Could you check a few things on this model? Use its own coordinates, in mm. Face numbers are marked on the shaded views. A direction names the side the tool comes from. Coordinates: 2 decimals unless noted, no trailing zeros. Write each loop counter-clockwise with the first axis right and the second up, starting at its lowest first coordinate (ties: lowest second). Pieces come first, ordered by that corner, then holes. Notation, with made-up numbers: (31, 57) - (71, 57) arc R27 ccw to (71, 82) - close; hole circle Ø7 at (77.5, 48). An arc over 180 degrees is marked (long way). Answer as a JSON object with one key per item and string values. Group by question number.
1) If we section it at C-C (x = -1.75): Write out the boundary of the cut face in (y, z).
2) On a 3-axis mill with a long thin cutter (end or side, diameter ignored), from which of +Z, -Z, +X, -X, +Y, -Y can I reach the whole of each face in a straight line? I mean the marked faces 1, 2, 3, 4 and 5. Say none if no direction works.
3) If we section it at D-D (y = 10.5): Write out the boundary of the cut face in (x, z).
4) If we section it at A-A (y = 8): Write out the boundary of the cut face in (x, z), plus the area to 3 significant figures.
5) We'd pull the mould along X, two halves only. Please class the marked faces 6, 7, 8 and 9: released by +X, released by -X, zero draft, split by the parting line, or undercut.
6) Will these pins go through, and if not, where does the flat tip stop? pin 1 Ø3 at (y, z) = (8, 0) entering from +X; pin 2 Ø6.5 at (y, z) = (6.5, 1) entering from +X; pin 3 Ø0.6 at (y, z) = (5.5, 7.5) entering from -X; pin 4 Ø4.5 at (y, z) = (-1.5, -1.5) entering from +X.
7) Please list where these lines run through material, in increasing order: line 1 along Y through (x, z) = (-14.05, 0); line 2 along X through (y, z) = (15.5, 7.5); line 3 along Z through (x, y) = (-11.8, 8).
8) If we section it at B-B (z = 0): Write out the boundary of the cut face in (x, y), plus the area to 3 significant figures.
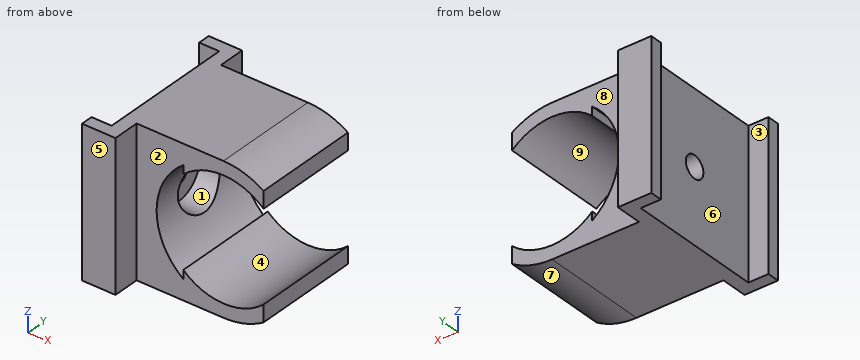
Autodesk Fusion 360 part; units mm, degrees
cylinder "CylinderPrimitive1" add diameter 18.5 height 80 placed x (1, 0, 0) y (0, 0, -1) z (0, 1, 0) at (0, 0, 0) makes body 1
sketch "Sketch2" plane through (0, 0, 0) normal (0, 1, 0) x (1, 0, 0)
  circle A0 centre (0, 0) radius 9
  line L0 (-23.395, 11) -> (16.2834, 11)
  line L1 (16.2834, 11) -> (16.2834, -11)
  line L2 (16.2834, -11) -> (-23.395, -11)
  line L3 (-23.395, -11) -> (-23.395, 11)
  circle A1 centre (0, 0) radius 10
  line L4 (0, 17.0641) -> (0, -18.6824) construction
  line L5 (-36.3056, 0) -> (26.2246, 0) construction
  line L6 (0, 9) -> (13.2349, 9)
  line L7 (13.2349, 9) -> (13.2349, -9)
  line L8 (13.2349, -9) -> (0, -9)
  line L9 (0, -9) -> (0, 9)
  line L10 (6, 8) -> (6, -8)
  circle A2 centre (0, 0) radius 11
  line L11 (6, 8) -> (6, 11)
  line L12 (6, -8) -> (6, -11)
  line L13 (-13, 11) -> (-18, 11)
  line L14 (-18, 11) -> (-18, -11)
  line L15 (-18, -11) -> (-13, -11)
  line L16 (-13, -11) -> (-13, 11)
  line L17 (-6, 8) -> (-6, -8)
  line L18 (-6, -8) -> (-6, -11)
  line L19 (-6, 8) -> (-6, 11)
  dimension "d3" = 18
  dimension "d4" = 11
  dimension "d5" = 11
  dimension "d6" = 1
  dimension "d7" = 6
  dimension "d8" = 2
  dimension "d9" = 5
  dimension "d10" = 13
extrude "Extrude1" add sketch "Sketch2" along normal blind 16 separate body contours A0 A1 L6 L10 | A0 A1 L8 L10 | A0 A1 L6 L17 | A1 L6 L11 | A0 A1 L8 L17 | A1 L8 L12 | A1 L6 A2 L11 L19 | A1 L8 A2 L12 L18 | A1 A2 L18 L19 | L0 A2 L19 | L0 L2 A2 L16 L18 L19 | L2 A2 L18 | L0 L2 L13 L14 L15 L16 makes body 2
sketch "Sketch3" plane through (-18, 0, 0) normal (-1, 0, 0) x (0, 0, 1)
  line L0 (-11, 0) -> (11, 0)
  line L1 (11, 0) -> (11, 16)
  line L2 (11, 16) -> (-11, 16)
  line L3 (-11, 16) -> (-11, 0)
  line L4 (11, 16) -> (-11, 0)
  line L5 (-11, 16) -> (11, 0)
  line L6 (-14, 18.2) -> (14, 18.2)
  line L7 (14, 18.2) -> (14, -2.2)
  line L8 (14, -2.2) -> (-14, -2.2)
  line L9 (-14, -2.2) -> (-14, 18.2)
  point P0 (0, 8)
  dimension "d21" = 10.2
  dimension "d22" = 10.2
  dimension "d23" = 14
  dimension "d24" = 14
hole "Hole1" at (-18, 8, 0) direction (1, 0, 0) diameter 3.332 end through all bodies 1 2
extrude "Extrude2" add sketch "Sketch2" along normal blind 20 and the other way blind 4 contours L0 L2 L13 L14 L15 L16 bodies 2
extrude "Extrude3" cut sketch "Sketch3" against normal blind 3 contours L0 L4 L5 | L3 L4 L5 | L1 L4 L5 | L2 L4 L5 | L6 L7 L8 L9 bodies 2
hole "Hole2" at (-18, 8, 0) direction (1, 0, 0) diameter 3.332 end through all bodies 1 2
ref_plane "WorkPlane1" through (-9, 0, 0) normal (1, 0, 0) x (0, 1, 0)
sketch "Sketch4" plane through (-9, 0, 0) normal (1, 0, 0) x (0, 0, -1)
  point P0 (0, 8)
hole "Hole3" at (-9, 8, 0) direction (-1, 0, 0) diameter 8 depth 4 tip angle 180 bodies 2
hidden bodies 1
Here are the results:
{
 "1": {"outline": "(0, -11) - (16, -11) - (16, -8.83) - (0, -8.83) - close; (0, 8.83) - (16, 8.83) - (16, 11) - (0, 11) - close"},
 "2": {"face 1": "+X", "face 2": "+Z, -Z, +X, -Y", "face 3": "+Z, -Z, -X", "face 4": "+Y, -Y", "face 5": "+Z, -Z, +X, -X, -Y"},
 "3": {"outline": "(-15, -11) - (0, -11) arc R11 ccw to (6, -9.22) - (6, -6.71) arc R9 cw to (-6, -6.71) - (-6, -8) arc R10 cw to (-9.5, -3.12) - (-13, -3.12) - (-13, 3.12) - (-9.5, 3.12) arc R10 cw to (-6, 8) - (-6, 6.71) arc R9 cw to (6, 6.71) - (6, 9.22) arc R11 ccw to (0, 11) - (-15, 11) - close"},
 "4": {"outline": "(-15, -11) - (0, -11) arc R11 ccw to (6, -9.22) - (6, -6.71) arc R9 cw to (-6, -6.71) - (-6, -8) arc R10 cw to (-9.17, -4) - (-13, -4) - (-13, -1.67) - (-15, -1.67) - close; (-15, 1.67) - (-13, 1.67) - (-13, 4) - (-9.17, 4) arc R10 cw to (-6, 8) - (-6, 6.71) arc R9 cw to (6, 6.71) - (6, 9.22) arc R11 ccw to (0, 11) - (-15, 11) - close", "area": "179 mm²"},
 "5": {"face 6": "released by -X", "face 7": "released by +X", "face 8": "zero draft", "face 9": "undercut"},
 "6": {"pin 1": "passes through", "pin 2": "stops at x = -9.05", "pin 3": "stops at x = -15", "pin 4": "stops at x = -9.48"},
 "7": {"line 1": "y = -4 to 6.33, 9.67 to 20", "line 2": "x = -15 to -6.61, -6 to -4.97, 4.97 to 6", "line 3": "z = -11 to -4, 4 to 11"},
 "8": {"outline": "(-18, -4) - (-13, -4) - (-13, 0) - (-10, 0) - (-10, 4) - (-13, 4) - (-13, 6.33) - (-15, 6.33) - (-15, -2.2) - (-18, -2.2) - close; (-18, 18.2) - (-15, 18.2) - (-15, 9.67) - (-13, 9.67) - (-13, 12) - (-10, 12) - (-10, 16) - (-13, 16) - (-13, 20) - (-18, 20) - close", "area": "76.1 mm²"}
}
